The model under review builds one solid part; all positions refer to its coordinate system, in mm. Face numbers are marked on the shaded views. A direction names the side the tool comes from. Give positions to 0.01 mm unless a question says otherwise; leave off trailing zeros. Order: outer loops, then holes, each group sorted by start corner. A loop starts at its lowest first (then second) coordinate and runs counter-clockwise, first axis right, second up.
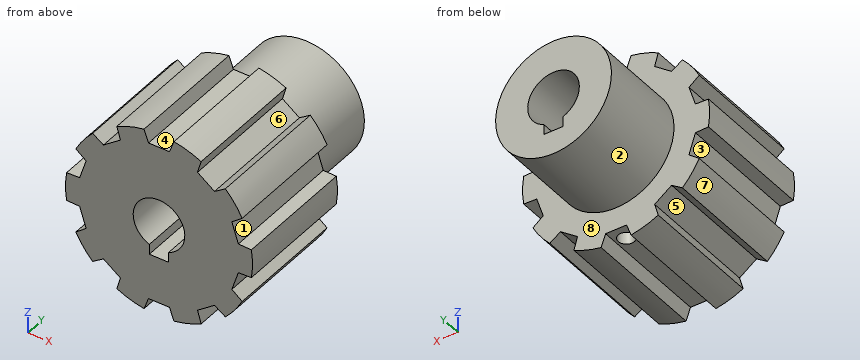
```python
from build123d import *

# Parameters (mm, degrees)
BOSS_EXTRUDE1_DEPTH       = 19
SKETCH3_R                 = 4.01
CUT_EXTRUDE1_DEPTH        = 29.952983186
SKETCH4_W                 = 3
SKETCH4_H                 = 4.35070692
CUT_EXTRUDE2_DEPTH        = 29.952983186
BOSS_EXTRUDE2_START       = 14
SKETCH5_R                 = 9
BOSS_EXTRUDE2_DEPTH       = 14
M3X0_5_TAPPED_HOLE1_D     = 2.5
M3X0_5_TAPPED_HOLE1_DEPTH = 10
M3X0_5_TAPPED_HOLE1_TIP   = 0.751075774


with BuildPart() as part:
    # Sketch2 → Boss-Extrude1 (new body)
    with BuildSketch(Plane(origin=(0, 0, 0), x_dir=(1, 0, 0), z_dir=(0, 1, 0))):
        with BuildLine():
            Line((7.335535963, -10.343914335), (9.974123377, -8.426868365))
            Line((9.974123377, -8.426868365), (11.654796972, -9.560497019))
            ThreePointArc((11.654796972, -9.560497019), (13.098043776, -7.864477351), (14.265066544, -5.967769174))
            Line((14.265066544, -5.967769174), (12.667564922, -4.719664118))
            Line((12.667564922, -4.719664118), (13.675415632, -1.617818581))
            Line((13.675415632, -1.617818581), (15.701439337, -1.547068275))
            ThreePointArc((15.701439337, -1.547068275), (15.87215518, 0.673359646), (15.701439337, 2.893787567))
            Line((15.701439337, 2.893787567), (13.675415632, 2.964537874))
            Line((13.675415632, 2.964537874), (12.667564922, 6.066383411))
            Line((12.667564922, 6.066383411), (14.265066544, 7.314488466))
            ThreePointArc((14.265066544, 7.314488466), (13.098043776, 9.211196644), (11.654796972, 10.907216312))
            Line((11.654796972, 10.907216312), (9.974123377, 9.773587658))
            Line((9.974123377, 9.773587658), (7.335535963, 11.690633627))
            Line((7.335535963, 11.690633627), (7.894324179, 13.639359722))
            ThreePointArc((7.894324179, 13.639359722), (5.835325832, 14.487870099), (3.670819293, 15.011659646))
            Line((3.670819293, 15.011659646), (2.977455996, 13.106659646))
            Line((2.977455996, 13.106659646), (-0.284017411, 13.106659646))
            Line((-0.284017411, 13.106659646), (-0.977380707, 15.011659646))
            ThreePointArc((-0.977380707, 15.011659646), (-3.141887247, 14.487870099), (-5.200885594, 13.639359722))
            Line((-5.200885594, 13.639359722), (-4.642097378, 11.690633627))
            Line((-4.642097378, 11.690633627), (-7.280684791, 9.773587658))
            Line((-7.280684791, 9.773587658), (-8.961358387, 10.907216312))
            ThreePointArc((-8.961358387, 10.907216312), (-10.40460519, 9.211196644), (-11.571627958, 7.314488466))
            Line((-11.571627958, 7.314488466), (-9.974126336, 6.066383411))
            Line((-9.974126336, 6.066383411), (-10.981977046, 2.964537874))
            Line((-10.981977046, 2.964537874), (-13.008000751, 2.893787567))
            ThreePointArc((-13.008000751, 2.893787567), (-13.178716594, 0.673359646), (-13.008000751, -1.547068275))
            Line((-13.008000751, -1.547068275), (-10.981977046, -1.617818581))
            Line((-10.981977046, -1.617818581), (-9.974126336, -4.719664118))
            Line((-9.974126336, -4.719664118), (-11.571627958, -5.967769174))
            ThreePointArc((-11.571627958, -5.967769174), (-10.40460519, -7.864477351), (-8.961358387, -9.560497019))
            Line((-8.961358387, -9.560497019), (-7.280684791, -8.426868365))
            Line((-7.280684791, -8.426868365), (-4.642097378, -10.343914335))
            Line((-4.642097378, -10.343914335), (-5.200885594, -12.292640429))
            ThreePointArc((-5.200885594, -12.292640429), (-3.141887247, -13.141150806), (-0.977380707, -13.664940354))
            Line((-0.977380707, -13.664940354), (-0.284017411, -11.759940354))
            Line((-0.284017411, -11.759940354), (2.977455996, -11.759940354))
            Line((2.977455996, -11.759940354), (3.670819293, -13.664940354))
            ThreePointArc((3.670819293, -13.664940354), (5.835325832, -13.141150806), (7.894324179, -12.292640429))
            Line((7.894324179, -12.292640429), (7.335535963, -10.343914335))
        make_face()
    extrude(amount=BOSS_EXTRUDE1_DEPTH)

    # Sketch3 → Cut-Extrude1 (cut, through all)
    with BuildSketch(Plane(origin=(0, 19, 0), x_dir=(1, 0, 0), z_dir=(0, 1, 0))):
        with Locations(Location((1.346719293, 0.673359646, 0), (0, 0, 270))):
            Circle(SKETCH3_R)
    extrude(amount=-CUT_EXTRUDE1_DEPTH, mode=Mode.SUBTRACT)

    # Sketch4 → Cut-Extrude2 (cut, through all)
    with BuildSketch(Plane(origin=(0, 19, 0), x_dir=(1, 0, 0), z_dir=(0, 1, 0))):
        with Locations((1.346719293, 3.788006186)):
            Rectangle(SKETCH4_W, SKETCH4_H)
    extrude(amount=-CUT_EXTRUDE2_DEPTH, mode=Mode.SUBTRACT)

    # Sketch5 → Boss-Extrude2 (add)
    with BuildSketch(Plane(origin=(0, 19, 0), x_dir=(1, 0, 0), z_dir=(0, 1, 0)).offset(BOSS_EXTRUDE2_START)):
        with Locations(Location((1.346719293, 0.673359646, 0), (0, 0, 270))):
            Circle(SKETCH5_R)
        with BuildLine():
            Line((2.846719293, 4.392243888), (2.846719293, 5.963359646))
            Line((2.846719293, 5.963359646), (-0.153280707, 5.963359646))
            Line((-0.153280707, 5.963359646), (-0.153280707, 4.392243888))
            ThreePointArc((-0.153280707, 4.392243888), (1.346719293, -3.336640354), (2.846719293, 4.392243888))
        make_face(mode=Mode.SUBTRACT)
    extrude(amount=-BOSS_EXTRUDE2_DEPTH)

    # M3x0.5 Tapped Hole1
    with Locations(Plane(origin=(1.346719293, 16.7, -13.106659646), x_dir=(-1, 0, 0), z_dir=(0, 0, -1))):
        with Locations((0, 0)):
            Hole(M3X0_5_TAPPED_HOLE1_D / 2, depth=M3X0_5_TAPPED_HOLE1_DEPTH)
            with Locations((0, 0, -(M3X0_5_TAPPED_HOLE1_DEPTH + M3X0_5_TAPPED_HOLE1_TIP / 2))):  # 118° drill point
                Cone(0, M3X0_5_TAPPED_HOLE1_D / 2, M3X0_5_TAPPED_HOLE1_TIP, mode=Mode.SUBTRACT)


solid = part.part
```
1. For the marked faces 1, 2, 3, 4 and 5, list the 3-axis set-ups (+Z, -Z, +X, -X, +Y, -Y) from which the entire face can be reached by the end or side of a thin tool; tool diameter is ignored.
2. Draft analysis for pull direction X (two halves, no side actions). For the marked faces 6, 7 and 8, state which applies: pulls with the +X half, pulls with the -X half, needs draft (parallel to the pull), parting line crosses it, or undercut.
3. Take a section at D-D (y = 21.5). Write out the cut boundary in (x, z).
4. Insertion check: pin 1 (12 mm diameter, centred on x = -9.5, y = 6, fed in from -Z); pin 2 (4 mm diameter, centred on x = -9.5, z = 9, fed in from +Y); pin 3 (0.5 mm diameter, centred on y = 8.5, z = -5.5, fed in from +X). Each pin has a flat end and moves straight along its axis. Give the tip position at first contact, or say it passes through.
5. Take a section at A-A (x = 4.25). Write out the cut boundary in (y, z).
6. Take a section at B-B (z = 2.5). Write out the cut boundary in (x, y), and give its area (3 significant figures).
7. To check wall thickness, follow line 1 (X direction, y = 18.5, z = -10.75); line 2 (Y direction, x = -10.25, z = 7.75); line 3 (X direction, y = 3.5, z = 1.25). State the ranges of each line that lie inside material, in increasing order.
8. Take a section at C-C (x = 13.25). Write out the cut boundary in (y, z), and give its area (3 significant figures).
Answer:
1. face 1: +X, +Y, -Y
1. face 2: +Y
1. face 3: -X, +Y, -Y
1. face 4: +Z, +Y, -Y
1. face 5: +Y, -Y
2. face 6: undercut
2. face 7: pulls with the -X half
2. face 8: needs draft
3. outline: circle Ø18 at (1.35, -0.67); hole (-0.15, -5.96) - (2.85, -5.96) - (2.85, -4.39) arc R4.01 ccw (long way) to (-0.15, -4.39) - close
4. pin 1: stops at z = -14.37
4. pin 2: stops at y = 19
4. pin 3: stops at x = 12.93
5. outline: (0, -14.91) - (19, -14.91) - (19, -9.19) - (33, -9.19) - (33, -3.44) - (0, -3.44) - close; (0, 2.09) - (33, 2.09) - (33, 7.85) - (19, 7.85) - (19, 13.56) - (0, 13.56) - close
6. outline: (-10.7, 0) - (-1.1, 0) - (-1.1, 33) - (-7.08, 33) - (-7.08, 19) - (-10.7, 19) - close; (3.8, 0) - (13.39, 0) - (13.39, 19) - (9.77, 19) - (9.77, 33) - (3.8, 33) - close
6. area: 532 mm2
7. line 1: x = -9.12 to -8.73, -5.94 to 8.63, 11.42 to 11.81
7. line 2: y = 0 to 19
7. line 3: x = -13.05 to -2.17, 4.87 to 15.74
8. outline: (0, -9) - (19, -9) - (19, -6.52) - (0, -6.52) - close; (0, -4.27) - (19, -4.27) - (19, 2.93) - (0, 2.93) - close; (0, 5.17) - (19, 5.17) - (19, 7.65) - (0, 7.65) - close
8. area: 231 mm2
